For this review, use the dimensioned drawing (mm, ordinates from the lowest corner) and the shaded views. A direction names the side the tool comes from. Round coordinates to 2 decimals unless told otherwise and drop trailing zeros. Order: outer loops, then holes, each group sorted by start corner. A loop starts at its lowest first (then second) coordinate and runs counter-clockwise, first axis right, second up. Notation, with made-up numbers: M 6,-12.75 L 45,-12.75 A30 cw 45,14.25 Z; hole C 48.25,28 d10. An arc over 180 degrees is marked long. Use a Markdown table: item, result. Add a question column.
1. For the marked faces 4, 5 and 6, list the 3-axis set-ups (+Z, -Z, +X, -X, +Y, -Y) from which the entire face can be reached by the end or side of a thin tool; tool diameter is ignored.
2. Consider section A-A on x = 52. State the section outline as (y, z) points.
3. Consider section D-D on x = 9.5. State the section outline as (y, z) points.
4. Insertion check: P1, Ø10, axis at y = 18, z = 3, coming from the +X side; P2, Ø5, axis at y = 16.5, z = 6.5, coming from the -X side; P3, Ø5, axis at y = 18.5, z = 11.5, coming from the +X side. Each pin has a flat end and moves straight along its axis. Give the tip position at first contact, or say it passes through.
5. The part is to be moulded in two halves that separate along Z. For the marked faces 1, 2 and 3, say which applies: +Z half, -Z half, draft (parallel to the pull), parting line (faces both ways), or undercut.
6. Consider section B-B on z = 8.5. Count the separate pieces of the cut face and the enclosed holes in it.
7. To check wall thickness, follow probe 1 along X at (y, z) = (7.5, 13.25) (1 decimal); probe 2 along X at (y, z) = (4.5, 6) (1 decimal); probe 3 along X at (y, z) = (21.5, 7.75). State the ranges of each line that lie inside material, in increasing order.
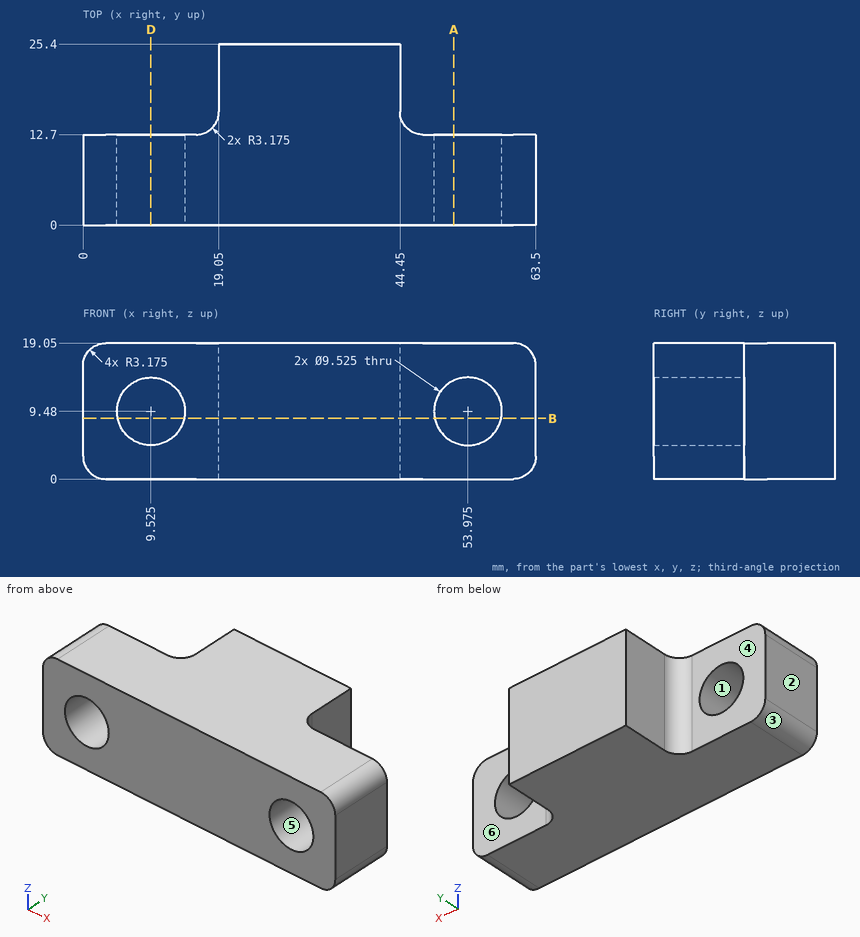
Answer block:
| question | item | result |
|---|---|---|
| 1 | face 4 | +Z, -Z, -X, +Y |
| 1 | face 5 | +Y, -Y |
| 1 | face 6 | +Z, -Z, +X, +Y |
| 2 | outline | M 0,0 L 12.7,0 L 12.7,5.15 L 0,5.15 Z; M 0,13.81 L 12.7,13.81 L 12.7,19.05 L 0,19.05 Z |
| 3 | outline | M 0,0 L 12.7,0 L 12.7,4.72 L 0,4.72 Z; M 0,14.24 L 12.7,14.24 L 12.7,19.05 L 0,19.05 Z |
| 4 | P1 | x = 46.28 |
| 4 | P2 | x = 18.44 |
| 4 | P3 | x = 44.45 |
| 5 | face 1 | undercut |
| 5 | face 2 | draft |
| 5 | face 3 | -Z half |
| 6 | separate pieces | 3 |
| 6 | enclosed holes | 0 |
| 7 | probe 1 | 0 to 6.6, 12.4 to 51.1, 56.9 to 63.5 |
| 7 | probe 2 | 0 to 6.3, 12.8 to 50.7, 57.2 to 63.5 |
| 7 | probe 3 | 19.05 to 44.45 |
